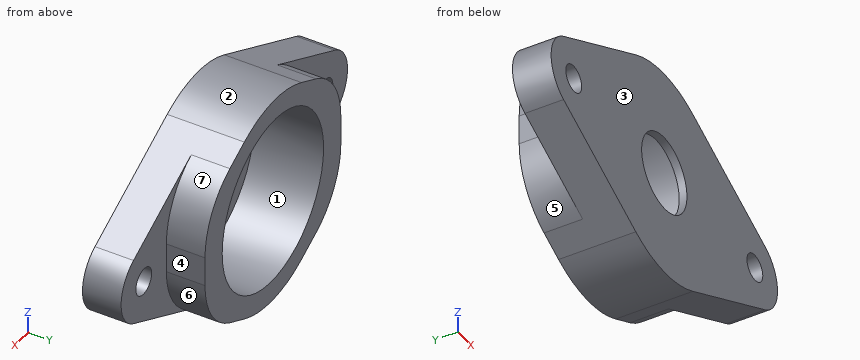
from build123d import *

# Parameters (mm, degrees)
SKETCH2_R               = 1.75
BOSS_EXTRUDE1_DEPTH     = 10
SKETCH3_R               = 11.2
CUT_EXTRUDE1_DEPTH      = 9
SKETCH4_W               = 10
SKETCH4_H               = 5
CUT_EXTRUDE2_DEPTH      = 15
CUT_EXTRUDE2_DEPTH_BACK = 15
FILLET1_R               = 10
SKETCH5_R               = 5
CUT_EXTRUDE3_DEPTH      = 10
CUT_EXTRUDE3_DEPTH_BACK = 2


with BuildPart() as part:
    # Sketch2 → Boss-Extrude1 (new body)
    with BuildSketch(Plane(origin=(0, 0, 0), x_dir=(1, 0, 0), z_dir=(0, 1, 0))):
        with BuildLine():
            Line((-22.25, 4.465142775), (-6.3, 12.50239977))
            ThreePointArc((-6.3, 12.50239977), (0, 14), (6.3, 12.50239977))
            Line((6.3, 12.50239977), (22.25, 4.465142775))
            ThreePointArc((22.25, 4.465142775), (25, 0), (22.25, -4.465142775))
            Line((22.25, -4.465142775), (6.3, -12.50239977))
            ThreePointArc((6.3, -12.50239977), (0, -14), (-6.3, -12.50239977))
            Line((-6.3, -12.50239977), (-22.25, -4.465142775))
            ThreePointArc((-22.25, -4.465142775), (-25, 0), (-22.25, 4.465142775))
        make_face()
        with Locations((-20, 0)):
            Circle(SKETCH2_R, mode=Mode.SUBTRACT)
        with Locations((20, 0)):
            Circle(SKETCH2_R, mode=Mode.SUBTRACT)
    extrude(amount=BOSS_EXTRUDE1_DEPTH)

    # Sketch3 → Cut-Extrude1 (cut)
    with BuildSketch(Plane(origin=(0, 10, 0), x_dir=(1, 0, 0), z_dir=(0, 1, 0))):
        Circle(SKETCH3_R)
    extrude(amount=-CUT_EXTRUDE1_DEPTH, mode=Mode.SUBTRACT)

    # Sketch4 → Cut-Extrude2 (cut, two sides)
    with BuildSketch(Plane.XY) as cut_extrude2_sk:
        with Locations((-20, 7.5)):
            Rectangle(SKETCH4_W, SKETCH4_H)
        with Locations((20, 7.5)):
            Rectangle(SKETCH4_W, SKETCH4_H)
    extrude(amount=CUT_EXTRUDE2_DEPTH, mode=Mode.SUBTRACT)
    extrude(cut_extrude2_sk.sketch, amount=-CUT_EXTRUDE2_DEPTH_BACK, mode=Mode.SUBTRACT)

    # Fillet1
    fillet1_edges = [part.edges().sort_by_distance(p)[0] for p in [
        (-15, 7.5, -8.118441409),
        (15, 7.5, -8.118441409),
        (-15, 7.5, 8.118441409),
        (15, 7.5, 8.118441409),
    ]]
    fillet(fillet1_edges, radius=FILLET1_R)

    # Sketch5 → Cut-Extrude3 (cut, two sides)
    with BuildSketch(Plane(origin=(0, 1, 0), x_dir=(1, 0, 0), z_dir=(0, 1, 0))) as cut_extrude3_sk:
        Circle(SKETCH5_R)
    extrude(amount=CUT_EXTRUDE3_DEPTH, mode=Mode.SUBTRACT)
    extrude(cut_extrude3_sk.sketch, amount=-CUT_EXTRUDE3_DEPTH_BACK, mode=Mode.SUBTRACT)


solid = part.part
For this review, take the finished solid that the model builds, in its own axes (mm). Face numbers are marked on the shaded views. A direction names the side the tool comes from. Round coordinates to 2 decimals unless told otherwise and drop trailing zeros. Order: outer loops, then holes, each group sorted by start corner. A loop starts at its lowest first (then second) coordinate and runs counter-clockwise, first axis right, second up. Notation, with made-up numbers: M 14,3.5 L 64,3.5 A17 ccw 64,33.5 Z; hole C 83,-5 d1. An arc over 180 degrees is marked long. Write each question's results on one line, items separated by ' | '. Start each with the question number.
1. Tool access review of the marked faces 4, 5, 6 and 7: name each direction out of +Z, -Z, +X, -X, +Y, -Y from which nothing blocks a thin tool from reaching the whole face with its end or side.
2. Add section A-A (x = 0). State the section outline as (y, z) points, then the cut area to 3 significant figures.
3. Add section B-B (y = 8). State the section outline as (x, z) points.
4. Clearance check with flat-ended pins moving along their axes: pin 1 Ø13.5 at (x, z) = (0, 0) entering from +Y; pin 2 Ø1.5 at (x, y) = (13, 8.5) entering from +Z; pin 3 Ø3 at (y, z) = (8, 0) entering from +X. State where each tip first meets the part, or that it passes through.
5. Add section C-C (z = 0). State the section outline as (x, y) points, then the cut area to 3 significant figures.
6. To check wall thickness, follow L1, parallel to X at y = 0.2, z = 0; L2, parallel to X at y = 1.7, z = 0; L3, parallel to Y at x = -4, z = 8.25. State the ranges of each line that lie inside material, in increasing order. Write a range as [from, to].
7. Draft analysis for pull direction Z (two halves, no side actions). For the marked faces 1, 2 and 3, state which applies: pulls with the +Z half, pulls with the -Z half, needs draft (parallel to the pull), parting line crosses it, or undercut.
8. Add section D-D (y = 2.5). State the section outline as (x, z) points.
Output values:
1) face 4: +Z, -Z, +X, +Y | face 5: -Z, -X, +Y | face 6: -Z, +X, +Y | face 7: +Z, +X, +Y
2) outline: M 0,-14 L 10,-14 L 10,-11.2 L 1,-11.2 L 1,-5 L 0,-5 Z; M 0,5 L 1,5 L 1,11.2 L 10,11.2 L 10,14 L 0,14 Z | area: 68.4 mm^2
3) outline: M -15,-1.96 A10 ccw -9.5,-10.89 L -6.3,-12.5 A14 ccw 6.3,-12.5 L 9.5,-10.89 A10 ccw 15,-1.96 L 15,1.96 A10 ccw 9.5,10.89 L 6.3,12.5 A14 ccw -6.3,12.5 L -9.5,10.89 A10 ccw -15,1.96 Z; hole C 0,0 d22.4
4) pin 1: y = 1 | pin 2: z = 8.85 | pin 3: x = 15
5) outline: M -25,0 L -21.75,0 L -21.75,5 L -25,5 Z; M -18.25,0 L -5,0 L -5,1 L -11.2,1 L -11.2,10 L -15,10 L -15,5 L -18.25,5 Z; M 5,0 L 18.25,0 L 18.25,5 L 15,5 L 15,10 L 11.2,10 L 11.2,1 L 5,1 Z; M 21.75,0 L 25,0 L 25,5 L 21.75,5 Z | area: 153 mm^2
6) L1: [-25, -21.75], [-18.25, -5], [5, 18.25], [21.75, 25] | L2: [-25, -21.75], [-18.25, -11.2], [11.2, 18.25], [21.75, 25] | L3: [0, 1]
7) face 1: undercut | face 2: pulls with the +Z half | face 3: needs draft
8) outline: M -22.25,-4.47 L -6.3,-12.5 A14 ccw 6.3,-12.5 L 22.25,-4.47 A5 ccw 22.25,4.47 L 6.3,12.5 A14 ccw -6.3,12.5 L -22.25,4.47 A5 ccw Z; hole C -20,0 d3.5; hole C 0,0 d22.4; hole C 20,0 d3.5
